```python
from build123d import *

# Parameters (mm, degrees)
SKETCH1_W           = 106
SKETCH1_H           = 60
BOSS_EXTRUDE1_DEPTH = 10
SKETCH2_W           = 10
SKETCH2_H           = 60
BOSS_EXTRUDE2_DEPTH = 55
SKETCH3_W           = 30
SKETCH3_H           = 15
BOSS_EXTRUDE3_DEPTH = 20
SKETCH4_W           = 60
SKETCH4_H           = 15
BOSS_EXTRUDE4_DEPTH = 20
SKETCH5_R           = 4.5
CUT_EXTRUDE1_DEPTH  = 66
SKETCH6_R           = 6.5
CUT_EXTRUDE2_DEPTH  = 6.6
SKETCH7_R           = 3.3
CUT_EXTRUDE3_DEPTH  = 9.4


with BuildPart() as part:
    # Sketch1 → Boss-Extrude1 (new body)
    with BuildSketch(Plane(origin=(0, 0, 0), x_dir=(1, 0, 0), z_dir=(0, 1, 0))):
        Rectangle(SKETCH1_W, SKETCH1_H)
    extrude(amount=BOSS_EXTRUDE1_DEPTH)

    # Sketch2 → Boss-Extrude2 (add)
    with BuildSketch(Plane.XZ):
        with Locations((-48, 0)):
            Rectangle(SKETCH2_W, SKETCH2_H)
        with Locations((48, 0)):
            Rectangle(SKETCH2_W, SKETCH2_H)
    extrude(amount=BOSS_EXTRUDE2_DEPTH)

    # Sketch3 → Boss-Extrude3 (add)
    with BuildSketch(Plane(origin=(53, 0, 0), x_dir=(0, 0, -1), z_dir=(1, 0, 0))):
        with Locations((-15, -47.5)):
            Rectangle(SKETCH3_W, SKETCH3_H)
    extrude(amount=BOSS_EXTRUDE3_DEPTH)

    # Sketch4 → Boss-Extrude4 (add)
    with BuildSketch(Plane.ZY.offset(53)):
        with Locations((0, -47.5)):
            Rectangle(SKETCH4_W, SKETCH4_H)
    extrude(amount=BOSS_EXTRUDE4_DEPTH)

    # Sketch5 → Cut-Extrude1 (cut, through all)
    with BuildSketch(Plane(origin=(0, 10, 0), x_dir=(1, 0, 0), z_dir=(0, 1, 0))):
        with Locations((-32, 21)):
            Circle(SKETCH5_R)
        with Locations((32, 21)):
            Circle(SKETCH5_R)
        with Locations((32, -21)):
            Circle(SKETCH5_R)
        with Locations((-32, -21)):
            Circle(SKETCH5_R)
    extrude(amount=-CUT_EXTRUDE1_DEPTH, mode=Mode.SUBTRACT)

    # Sketch6 → Cut-Extrude2 (cut)
    with BuildSketch(Plane(origin=(0, -40, 0), x_dir=(1, 0, 0), z_dir=(0, 1, 0))):
        with Locations((63, -20)):
            Circle(SKETCH6_R)
        with Locations((-63, 20)):
            Circle(SKETCH6_R)
        with Locations((-63, -20)):
            Circle(SKETCH6_R)
    extrude(amount=-CUT_EXTRUDE2_DEPTH, mode=Mode.SUBTRACT)

    # Sketch7 → Cut-Extrude3 (cut, through all)
    with BuildSketch(Plane(origin=(0, -46.6, 0), x_dir=(1, 0, 0), z_dir=(0, 1, 0))):
        with Locations((-63, 20)):
            Circle(SKETCH7_R)
        with Locations((-63, -20)):
            Circle(SKETCH7_R)
        with Locations((63, -20)):
            Circle(SKETCH7_R)
    extrude(amount=-CUT_EXTRUDE3_DEPTH, mode=Mode.SUBTRACT)


solid = part.part
```
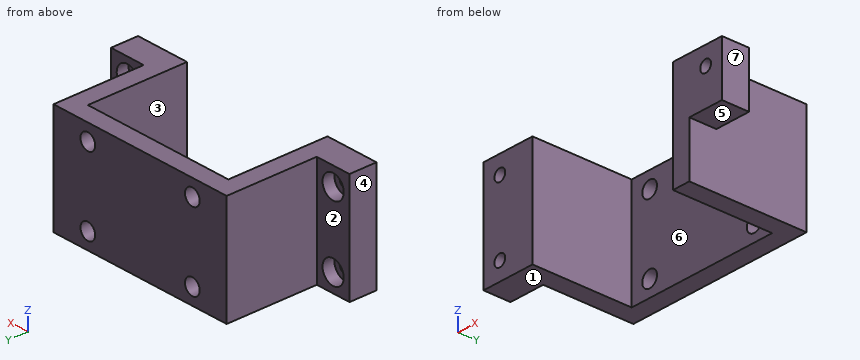
Check sheet for the modelled part. Datum: model origin and axes. Units: mm. Face numbers are marked on the shaded views. A direction names the side the tool comes from. Round coordinates to 2 decimals unless told otherwise and drop trailing zeros. Write each loop counter-clockwise with the first axis right and the second up, starting at its lowest first coordinate (ties: lowest second). Pieces come first, ordered by that corner, then holes. Notation, with made-up numbers: M -6.5,71 L -2.5,71 A4 ccw -2.5,76 Z; hole C 83.5,-17.75 d10. An arc over 180 degrees is marked long. Write item = value, one per line. Start each with the question number.
1. Gauge pin test, flat ends, axial feed: pin 1 (10 mm diameter, centred on y = -30, z = 12, fed in from +X); pin 2 (10.5 mm diameter, centred on x = -65, z = -19, fed in from +Y); pin 3 (3 mm diameter, centred on x = 9.5, z = 18, fed in from -Y). Record the tip position at first contact, or that the pin passes through.
2. Section check C-C, the plane x = 63. Record the cut outline in (y, z), then the cut area to 3 significant figures.
3. Release check for a two-part mould opening along X. For the marked faces 4, 5, 6 and 7 record: pulls with the +X half, pulls with the -X half, needs draft (parallel to the pull), parting line crosses it, or undercut.
4. Tool access check on the marked faces 1, 2 and 3. Record the directions out of +Z, -Z, +X, -X, +Y, -Y that give a thin tool (end or side, any length) a straight path to the whole face; none if there is none.
5. Section check B-B, the plane x = -63. Record the cut outline in (y, z).
6. Section check D-D, the plane z = 9.5. Record the cut outline in (x, y), then the cut area to 3 significant figures.
7. Scan lines: line 1 (X direction, y = 7, z = 21); line 2 (Z direction, x = -32, y = 5); line 3 (X direction, y = -52.75, z = 20). Record each from-to range of solid material in increasing order. Write a range as [from, to].
8. Section check A-A, the plane y = -33.5. Record the cut outline in (x, z).
Results found:
q1.pin_1 = 53
q1.pin_2 = -40
q1.pin_3 = 0
q2.outline = M -55,0 L -40,0 L -40,13.5 L -46.6,13.5 L -46.6,16.7 L -55,16.7 Z; M -55,23.3 L -46.6,23.3 L -46.6,26.5 L -40,26.5 L -40,30 L -55,30 Z
q2.area = 309 mm^2
q3.face_4 = pulls with the -X half
q3.face_5 = needs draft
q3.face_6 = undercut
q3.face_7 = pulls with the +X half
q4.face_1 = -Z, +X, -X, +Y, -Y
q4.face_2 = +Z, -Z, -X, +Y
q4.face_3 = +Z, -Z, -Y
q5.outline = M -55,-30 L -40,-30 L -40,-26.5 L -46.6,-26.5 L -46.6,-23.3 L -55,-23.3 Z; M -55,-16.7 L -46.6,-16.7 L -46.6,-13.5 L -40,-13.5 L -40,13.5 L -46.6,13.5 L -46.6,16.7 L -55,16.7 Z; M -55,23.3 L -46.6,23.3 L -46.6,26.5 L -40,26.5 L -40,30 L -55,30 Z
q6.outline = M -73,-55 L -43,-55 L -43,0 L 43,0 L 43,-55 L 73,-55 L 73,-40 L 53,-40 L 53,10 L -53,10 L -53,-40 L -73,-40 Z
q6.area = 2,760 mm^2
q7.line_1 = [-53, -36.5], [-27.5, 27.5], [36.5, 53]
q7.line_2 = [-30, -25.5], [-16.5, 16.5], [25.5, 30]
q7.line_3 = [-73, -66.3], [-59.7, -43], [43, 59.7], [66.3, 73]
q8.outline = M -53,-30 L -43,-30 L -43,30 L -53,30 Z; M 43,-30 L 53,-30 L 53,30 L 43,30 Z
